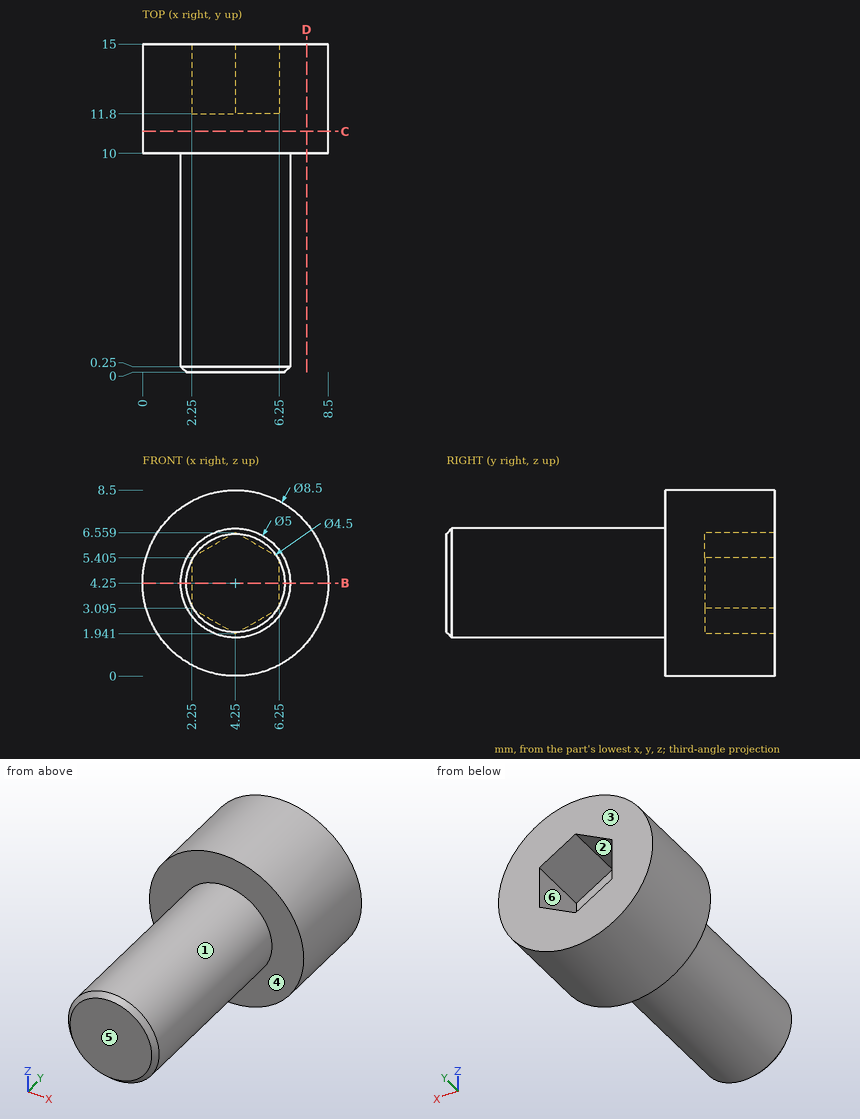
Could you check a few things on this drawing? It's one solid part, dimensions in mm from its lowest x, y, z. A direction names the side the tool comes from. Round coordinates to 2 decimals unless told otherwise and drop trailing zeros. Write each loop counter-clockwise with the first axis right and the second up, starting at its lowest first coordinate (ties: lowest second). Pieces come first, ordered by that corner, then holes.
Q1. If we mould it in two halves opening along Z, with no side actions, what happens to the marked faces 1, 2 and 3? For each: +Z half, -Z half, draft (parallel to the pull), parting line (faces both ways), or undercut.
Q2. Will these pins go through, and if not, where does the flat tip stop? P1, Ø1, axis at y = 11, z = 6.5, coming from the -X side; P2, Ø3, axis at x = 4.5, y = 3.5, coming from the -Z side; P3, Ø0.7, axis at y = 13.5, z = 3.5, coming from the -X side.
Q3. If we section it at B-B on z = 4.25: Write out the boundary of the cut face in (x, y).
Q4. Which directions (+Z, -Z, +X, -X, +Y, -Y) give clear straight access to the entire face, cutting with the end or side of a thin tool? Please do the marked faces 4, 5 and 6.
Q5. If we section it at C-C on y = 11: Write out the boundary of the cut face in (x, z).
Q6. Please list where these lines run through material, in increasing order: probe 1 along Y at (x, z) = (3.75, 4); probe 2 along X at (y, z) = (14.5, 6) (1 decimal); probe 3 along Y at (x, z) = (1, 2.25).
Q7. If we section it at D-D on x = 7.5: Write out the boundary of the cut face in (y, z).
Answer below:
1. face 1: parting line
1. face 2: undercut
1. face 3: draft
2. P1: stops at x = 0.38
2. P2: stops at z = 1.75
2. P3: stops at x = 0.02
3. outline: (0, 10) - (1.75, 10) - (1.75, 0.25) - (2, 0) - (6.5, 0) - (6.75, 0.25) - (6.75, 10) - (8.5, 10) - (8.5, 15) - (6.25, 15) - (6.25, 11.8) - (2.25, 11.8) - (2.25, 15) - (0, 15) - close
4. face 4: -Y
4. face 5: +Z, -Z, +X, -X, -Y
4. face 6: +Y
5. outline: circle Ø8.5 at (4.25, 4.25)
6. probe 1: y = 0 to 11.8
6. probe 2: x = 0.4 to 3.3, 5.2 to 8.1
6. probe 3: y = 10 to 15
7. outline: (10, 1.51) - (15, 1.51) - (15, 6.99) - (10, 6.99) - close
